The listing builds one solid part. Answer for the finished solid, in the listing's coordinates (mm). Face numbers are marked on the shaded views. A direction names the side the tool comes from. Coordinates: 2 decimals unless noted, no trailing zeros. Write each loop counter-clockwise with the first axis right and the second up, starting at its lowest first coordinate (ties: lowest second). Pieces come first, ordered by that corner, then holes.
from build123d import *

# Parameters (mm, degrees)
CROQUIS1_W              = 60.5
CROQUIS1_H              = 54.5
SALIENTE_EXTRUIR1_DEPTH = 25
CROQUIS2_W              = 56.9
CROQUIS2_H              = 50.9
CORTAR_EXTRUIR1_DEPTH   = 15
CROQUIS3_R              = 2.1
CORTAR_EXTRUIR2_DEPTH   = 5
CORTAR_EXTRUIR3_DEPTH   = 5
CORTAR_EXTRUIR4_DEPTH   = 1.8
CORTAR_EXTRUIR6_START   = -1.8
CORTAR_EXTRUIR6_DEPTH   = 60.5
CROQUIS10_W             = 6
CROQUIS10_H             = 6
CROQUIS10_R             = 1.6
SALIENTE_EXTRUIR2_DEPTH = 3
CROQUIS11_W             = 58.5
CROQUIS11_H             = 52.5
CORTAR_EXTRUIR7_DEPTH   = 15
CORTAR_EXTRUIR8_START   = -9.8
CROQUIS13_W             = 33.95
CROQUIS13_H             = 0.3
CORTAR_EXTRUIR8_DEPTH   = 9.8
CORTAR_EXTRUIR9_START   = -15
CROQUIS14_W             = 50.75
CROQUIS14_H             = 1
CORTAR_EXTRUIR9_DEPTH   = 15
SALIENTE_EXTRUIR3_DEPTH = 15.3
CROQUIS17_R             = 4
CROQUIS17_R_2           = 4.75
CORTAR_EXTRUIR10_DEPTH  = 1


with BuildPart() as part:
    # Croquis1 → Saliente-Extruir1 (new body)
    with BuildSketch(Plane.XY):
        with Locations((-43.305557703, 3.094674556)):
            Rectangle(CROQUIS1_W, CROQUIS1_H)
    extrude(amount=SALIENTE_EXTRUIR1_DEPTH)

    # Croquis2 → Cortar-Extruir1 (cut)
    with BuildSketch(Plane.XY.offset(25)):
        with Locations((-43.305557703, 3.094674556)):
            Rectangle(CROQUIS2_W, CROQUIS2_H)
    extrude(amount=-CORTAR_EXTRUIR1_DEPTH, mode=Mode.SUBTRACT)

    # Croquis3 → Cortar-Extruir2 (cut)
    with BuildSketch(Plane.XY.offset(10)):
        with Locations((-68.955557703, 25.744674556)):
            Circle(CROQUIS3_R)
        with Locations((-55.855557703, -19.355325444)):
            Circle(CROQUIS3_R)
        with Locations((-30.755557703, -19.355325444)):
            Circle(CROQUIS3_R)
        with Locations((-17.655557703, 25.744674556)):
            Circle(CROQUIS3_R)
        Polygon((-71.755557703, 20.544674556), (-71.755557703, -22.355325444), (-59.855557703, -22.355325444), (-59.855557703, -14.355325444), (-51.855557703, -14.355325444), (-51.855557703, -22.355325444), (-34.755557703, -22.355325444), (-34.755557703, -14.355325444), (-26.755557703, -14.355325444), (-26.755557703, -22.355325444), (-14.855557703, -22.355325444), (-14.855557703, 20.544674556), (-22.855557703, 20.544674556), (-22.855557703, 28.544674556), (-63.755557703, 28.544674556), (-63.755557703, 20.544674556), align=None)
    extrude(amount=-CORTAR_EXTRUIR2_DEPTH, mode=Mode.SUBTRACT)

    # Croquis5 → Cortar-Extruir3 (cut)
    with BuildSketch(Plane(origin=(0, -22.355325444, 0), x_dir=(1, 0, 0), z_dir=(0, 1, 0))):
        with BuildLine():
            Line((-18.605557703, -18), (-18.605557703, -25))
            Line((-18.605557703, -25), (-26.105557703, -25))
            Line((-26.105557703, -25), (-26.105557703, -18))
            ThreePointArc((-26.105557703, -18), (-22.355557703, -14.25), (-18.605557703, -18))
        make_face()
        with BuildLine():
            Line((-39.605557703, -18), (-39.605557703, -25))
            Line((-39.605557703, -25), (-47.105557703, -25))
            Line((-47.105557703, -25), (-47.105557703, -18))
            ThreePointArc((-47.105557703, -18), (-43.355557703, -14.25), (-39.605557703, -18))
        make_face()
        with BuildLine():
            Line((-60.605557703, -18), (-60.605557703, -25))
            Line((-60.605557703, -25), (-68.105557703, -25))
            Line((-68.105557703, -25), (-68.105557703, -18))
            ThreePointArc((-68.105557703, -18), (-64.355557703, -14.25), (-60.605557703, -18))
        make_face()
    extrude(amount=-CORTAR_EXTRUIR3_DEPTH, mode=Mode.SUBTRACT)

    # Croquis6 → Cortar-Extruir4 (cut)
    with BuildSketch(Plane.XZ.offset(-28.544674556)):
        Polygon((-64.805557703, 17), (-21.805557703, 17), (-21.805557703, 10), (-22.855557703, 10), (-22.855557703, 5), (-30.855557703, 5), (-30.855557703, 10), (-64.805557703, 10), align=None)
    extrude(amount=-CORTAR_EXTRUIR4_DEPTH, mode=Mode.SUBTRACT)

    # Croquis9 → Cortar-Extruir6 (cut)
    with BuildSketch(Plane(origin=(-71.755557703, 0, 0), x_dir=(0, 0, -1), z_dir=(1, 0, 0)).offset(CORTAR_EXTRUIR6_START)):
        with BuildLine():
            Line((-10, 20.544674556), (-20, 20.544674556))
            ThreePointArc((-20, 20.544674556), (-22.5, 18.044674556), (-20, 15.544674556))
            Line((-20, 15.544674556), (-10, 15.544674556))
            ThreePointArc((-10, 15.544674556), (-7.5, 18.044674556), (-10, 20.544674556))
        make_face()
        with BuildLine():
            Line((-10, 10.544674556), (-20, 10.544674556))
            ThreePointArc((-20, 10.544674556), (-22.5, 8.044674556), (-20, 5.544674556))
            Line((-20, 5.544674556), (-10, 5.544674556))
            ThreePointArc((-10, 5.544674556), (-7.5, 8.044674556), (-10, 10.544674556))
        make_face()
        with BuildLine():
            Line((-10, 0.544674556), (-20, 0.544674556))
            ThreePointArc((-20, 0.544674556), (-22.5, -1.955325444), (-20, -4.455325444))
            Line((-20, -4.455325444), (-10, -4.455325444))
            ThreePointArc((-10, -4.455325444), (-7.5, -1.955325444), (-10, 0.544674556))
        make_face()
        with BuildLine():
            Line((-10, -9.455325444), (-20, -9.455325444))
            ThreePointArc((-20, -9.455325444), (-22.5, -11.955325444), (-20, -14.455325444))
            Line((-20, -14.455325444), (-10, -14.455325444))
            ThreePointArc((-10, -14.455325444), (-7.5, -11.955325444), (-10, -9.455325444))
        make_face()
    extrude(amount=CORTAR_EXTRUIR6_DEPTH, mode=Mode.SUBTRACT)

    # Croquis10 → Saliente-Extruir2 (add)
    with BuildSketch(Plane.XY.offset(25)):
        with Locations((-76.555557703, 27.344674556)):
            Rectangle(CROQUIS10_W, CROQUIS10_H)
        with Locations((-76.555557703, 27.344674556)):
            Circle(CROQUIS10_R, mode=Mode.SUBTRACT)
        with Locations((-10.055557703, 27.344674556)):
            Rectangle(CROQUIS10_W, CROQUIS10_H)
        with Locations((-10.055557703, 27.344674556)):
            Circle(CROQUIS10_R, mode=Mode.SUBTRACT)
        with Locations((-10.055557703, -21.155325444)):
            Rectangle(CROQUIS10_W, CROQUIS10_H)
        with Locations((-10.055557703, -21.155325444)):
            Circle(CROQUIS10_R, mode=Mode.SUBTRACT)
        with Locations((-76.555557703, -21.155325444)):
            Rectangle(CROQUIS10_W, CROQUIS10_H)
        with Locations((-76.555557703, -21.155325444)):
            Circle(CROQUIS10_R, mode=Mode.SUBTRACT)
    extrude(amount=-SALIENTE_EXTRUIR2_DEPTH)

    # Croquis11 → Cortar-Extruir7 (cut)
    with BuildSketch(Plane.XY.offset(25)):
        with Locations((-43.305557703, 3.094674556)):
            Rectangle(CROQUIS11_W, CROQUIS11_H)
    extrude(amount=-CORTAR_EXTRUIR7_DEPTH, mode=Mode.SUBTRACT)

    # Croquis13 → Cortar-Extruir8 (cut)
    with BuildSketch(Plane(origin=(0, 30.344674556, 0), x_dir=(1, 0, 0), z_dir=(0, 1, 0)).offset(CORTAR_EXTRUIR8_START)):
        with Locations((-47.830557703, -9.85)):
            Rectangle(CROQUIS13_W, CROQUIS13_H)
    extrude(amount=CORTAR_EXTRUIR8_DEPTH, mode=Mode.SUBTRACT)

    # Croquis14 → Cortar-Extruir9 (cut)
    with BuildSketch(Plane.XY.offset(25).offset(CORTAR_EXTRUIR9_START)):
        with Locations((-39.430557703, 29.844674556)):
            Rectangle(CROQUIS14_W, CROQUIS14_H)
    extrude(amount=CORTAR_EXTRUIR9_DEPTH, mode=Mode.SUBTRACT)

    # Croquis16 → Saliente-Extruir3 (add)
    with BuildSketch(Plane.XY.offset(25)):
        Polygon((-64.805557703, 30.344674556), (-64.805557703, 56.41412893), (-14.055557703, 56.41412893), (-14.055557703, 30.344674556), (-13.055557703, 30.344674556), (-13.055557703, 57.41412893), (-65.805557703, 57.41412893), (-65.805557703, 30.344674556), align=None)
    extrude(amount=-SALIENTE_EXTRUIR3_DEPTH)

    # Croquis17 → Cortar-Extruir10 (cut)
    with BuildSketch(Plane(origin=(0, 57.41412893, 0), x_dir=(1, 0, 0), z_dir=(0, 1, 0))):
        with Locations((-60.305557703, -17.35)):
            Circle(CROQUIS17_R)
        with Locations((-49.305557703, -17.35)):
            Circle(CROQUIS17_R)
        with Locations((-37.305557703, -17.35)):
            Circle(CROQUIS17_R_2)
        with Locations((-25.305557703, -17.35)):
            Circle(CROQUIS17_R)
    extrude(amount=-CORTAR_EXTRUIR10_DEPTH, mode=Mode.SUBTRACT)


solid = part.part
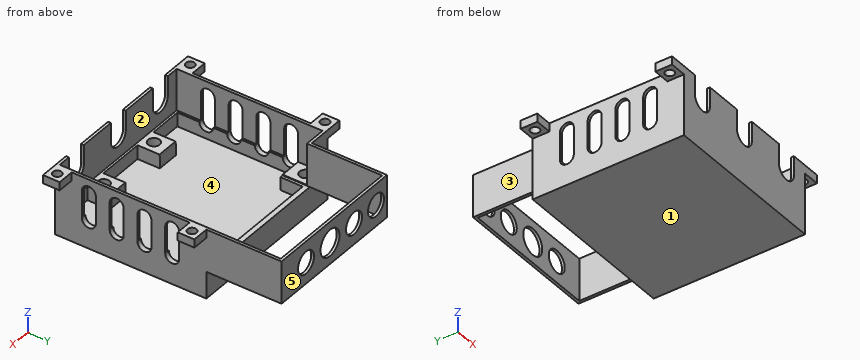
Q1. Determine the mould class of the marked faces 3, 4 and 5 for opening direction X: released by +X, released by -X, zero draft, split by the parting line, or undercut.
Answers below:
face 3: released by -X
face 4: undercut
face 5: zero draft
Q2. Find the intervals of material crossed by probe 1 along Y at (x, z) = (-14, 17.5); probe 2 along X at (y, z) = (56.8, 17.35); probe 3 along X at (y, z) = (27, 23.75), in increasing order.
Answers below:
probe 1: y = -24.16 to -14.46, -9.46 to -4.46, 0.54 to 5.54, 10.54 to 15.54, 20.54 to 57.41
probe 2: x = -65.81 to -64.31, -56.31 to -53.31, -45.31 to -42.06, -32.56 to -29.31, -21.31 to -13.06
probe 3: x = -79.56 to -78.12, -74.99 to -72.56, -14.06 to -11.62, -8.49 to -7.06
Q3. Given pin 1 (1 mm diameter, centred on x = -38, y = 0.5, fed in from +Z); pin 2 (0.5 mm diameter, centred on x = -73, z = 16, fed in from +Y); pin 3 (0.9 mm diameter, centred on x = -72, y = -6.5, fed in from +Z), each flat-ended and moving along its own axis, determine where each tip first touches the part or whether it passes through.
Answers below:
pin 1: stops at z = 5
pin 2: stops at y = 30.34
pin 3: stops at z = 10
Q4. The part is cut by section A-A, the plane y = 17. Write down the section's boundary in (x, z), then the cut area to 3 significant figures.
Answers below:
outline: (-73.56, 0) - (-13.06, 0) - (-13.06, 7.73) - (-14.86, 7.73) - (-14.86, 5) - (-71.76, 5) - (-71.76, 7.73) - (-73.56, 7.73) - close; (-73.56, 22.27) - (-72.56, 22.27) - (-72.56, 25) - (-73.56, 25) - close; (-14.06, 22.27) - (-13.06, 22.27) - (-13.06, 25) - (-14.06, 25) - close
area: 318 mm2
Q5. The part is cut by section B-B, the plane z = 16. State how many separate pieces and enclosed holes the cut face has, then the cut area to 3 significant figures.
Answers below:
separate pieces: 15
enclosed holes: 0
area: 189 mm2
Q6. Which of the six approach directions +Z, -Z, +X, -X, +Y, -Y give full straight-line access (tool end or side, diameter ignored) to the marked faces 1 and 2?
Answers below:
face 1: -Z, +X, -X, +Y, -Y
face 2: +Z
Q7. The part is cut by section C-C, the plane z = 4. Write down the section's boundary in (x, y).
Answers below:
outline: (-73.56, -24.16) - (-13.06, -24.16) - (-13.06, 30.34) - (-73.56, 30.34) - close
